from build123d import *

# Parameters (mm, degrees)
SKETCH1_R           = 25
SKETCH1_R_2         = 10
SKETCH1_R_3         = 4
SKETCH1_R_4         = 20
BOSS_EXTRUDE1_DEPTH = 17.5
SKETCH1_4_R         = 25
SKETCH1_4_R_2       = 20
BOSS_EXTRUDE2_DEPTH = 27.5
SKETCH2_R           = 20
CUT_EXTRUDE1_DEPTH  = 12.5
CUT_EXTRUDE2_DEPTH  = 55.083893922
SKETCH1_5_R         = 10
SKETCH1_5_R_2       = 6
BOSS_EXTRUDE3_DEPTH = 21.5
FILLET3_R           = 15
CUT_EXTRUDE3_DEPTH  = 12.5
FILLET1_R           = 7.5
FILLET2_R           = 1.5


with BuildPart() as part:
    # Sketch1 → Boss-Extrude1 (new body, symmetric)
    with BuildSketch(Plane(origin=(0, 0, 0), x_dir=(1, 0, 0), z_dir=(0, 1, 0))):
        with BuildLine():
            ThreePointArc((23.169245136, -48.74831039), (44.696355929, -24.926018406), (75, -14.314362055))
            Line((75, -14.314362055), (171.881275704, -5.838348723))
            ThreePointArc((171.881275704, -5.838348723), (170, 0), (171.881275704, 5.838348723))
            Line((171.881275704, 5.838348723), (75, 14.314362055))
            ThreePointArc((75, 14.314362055), (44.696355929, 24.926018406), (23.169245136, 48.74831039))
            ThreePointArc((23.169245136, 48.74831039), (24.030815541, 46.486476164), (24.323725422, 44.083893922))
            ThreePointArc((24.323725422, 44.083893922), (11.593351964, 34.463859578), (5.814713266, 49.337151209))
            ThreePointArc((5.814713266, 49.337151209), (-11.588137289, 35.664619361), (-33.70385172, 36.496791078))
            ThreePointArc((-33.70385172, 36.496791078), (-29.194535449, 32.814838368), (-27.5, 27.2453448))
            ThreePointArc((-27.5, 27.2453448), (-34.054404214, 17.857700278), (-45.125573936, 20.776139119))
            ThreePointArc((-45.125573936, 20.776139119), (-37.5, 0), (-45.125573936, -20.776139119))
            ThreePointArc((-45.125573936, -20.776139119), (-34.054404214, -17.857700278), (-27.5, -27.2453448))
            ThreePointArc((-27.5, -27.2453448), (-29.194535449, -32.814838368), (-33.70385172, -36.496791078))
            ThreePointArc((-33.70385172, -36.496791078), (-11.588137289, -35.664619361), (5.814713266, -49.337151209))
            ThreePointArc((5.814713266, -49.337151209), (11.593351964, -34.463859578), (24.323725422, -44.083893922))
            ThreePointArc((24.323725422, -44.083893922), (24.030815541, -46.486476164), (23.169245136, -48.74831039))
        make_face()
        Circle(SKETCH1_R, mode=Mode.SUBTRACT)
        with Locations((14.323725422, 44.083893922)):
            Circle(SKETCH1_R_2)
        with Locations((14.323725422, 44.083893922)):
            Circle(SKETCH1_R_3, mode=Mode.SUBTRACT)
        with Locations((-37.5, 27.2453448)):
            Circle(SKETCH1_R_2)
        with Locations((-37.5, 27.2453448)):
            Circle(SKETCH1_R_3, mode=Mode.SUBTRACT)
        with Locations((-37.5, -27.2453448)):
            Circle(SKETCH1_R_2)
        with Locations((-37.5, -27.2453448)):
            Circle(SKETCH1_R_3, mode=Mode.SUBTRACT)
        with Locations((14.323725422, -44.083893922)):
            Circle(SKETCH1_R_2)
        with Locations((14.323725422, -44.083893922)):
            Circle(SKETCH1_R_3, mode=Mode.SUBTRACT)
        Circle(SKETCH1_R)
        Circle(SKETCH1_R_4, mode=Mode.SUBTRACT)
    extrude(amount=BOSS_EXTRUDE1_DEPTH, both=True)

    # Sketch1_4 → Boss-Extrude2 (add, symmetric)
    with BuildSketch(Plane(origin=(0, 0, 0), x_dir=(1, 0, 0), z_dir=(0, 1, 0))):
        Circle(SKETCH1_4_R)
        Circle(SKETCH1_4_R_2, mode=Mode.SUBTRACT)
    extrude(amount=BOSS_EXTRUDE2_DEPTH, both=True)

    # Sketch2 → Cut-Extrude1 (cut, symmetric)
    with BuildSketch(Plane(origin=(0, 0, 0), x_dir=(1, 0, 0), z_dir=(0, 1, 0))):
        Circle(SKETCH2_R)
        with BuildLine():
            ThreePointArc((9.905954739, 28.31734558), (-30, 0), (9.905954739, -28.31734558))
            ThreePointArc((9.905954739, -28.31734558), (42.01613595, -19.285159783), (75, -14.314362055))
            ThreePointArc((75, -14.314362055), (44.696355929, -24.926018406), (23.169245136, -48.74831039))
            ThreePointArc((23.169245136, -48.74831039), (14.662831175, -54.078142632), (5.814713266, -49.337151209))
            ThreePointArc((5.814713266, -49.337151209), (-11.588137289, -35.664619361), (-33.70385172, -36.496791078))
            ThreePointArc((-33.70385172, -36.496791078), (-45.590169944, -33.123197323), (-45.125573936, -20.776139119))
            ThreePointArc((-45.125573936, -20.776139119), (-37.5, 0), (-45.125573936, 20.776139119))
            ThreePointArc((-45.125573936, 20.776139119), (-45.590169944, 33.123197323), (-33.70385172, 36.496791078))
            ThreePointArc((-33.70385172, 36.496791078), (-11.588137289, 35.664619361), (5.814713266, 49.337151209))
            ThreePointArc((5.814713266, 49.337151209), (14.662831175, 54.078142632), (23.169245136, 48.74831039))
            ThreePointArc((23.169245136, 48.74831039), (44.696355929, 24.926018406), (75, 14.314362055))
            ThreePointArc((75, 14.314362055), (42.01613595, 19.285159783), (9.905954739, 28.31734558))
        make_face()
    extrude(amount=CUT_EXTRUDE1_DEPTH, both=True, mode=Mode.SUBTRACT)

    # Sketch3 → Cut-Extrude2 (cut, symmetric)
    with BuildSketch(Plane.XY):
        with BuildLine():
            Line((171.881275704, 17.5), (171.881275704, 9.5))
            Line((171.881275704, 9.5), (119.899888641, 9.5))
            ThreePointArc((119.899888641, 9.5), (97.096380139, 11.515625954), (75, 17.5))
            Line((75, 17.5), (119.899888641, 17.5))
            Line((119.899888641, 17.5), (171.881275704, 17.5))
        make_face()
    cut_extrude2 = extrude(amount=CUT_EXTRUDE2_DEPTH, both=True, mode=Mode.SUBTRACT)

    # Mirror1: Cut-Extrude2 across plane
    add(cut_extrude2.mirror(Plane.ZX), mode=Mode.SUBTRACT)

    # Sketch1_5 → Boss-Extrude3 (add, symmetric)
    with BuildSketch(Plane(origin=(0, 0, 0), x_dir=(1, 0, 0), z_dir=(0, 1, 0))):
        with Locations((180, 0)):
            Circle(SKETCH1_5_R)
        with Locations((180, 0)):
            Circle(SKETCH1_5_R_2, mode=Mode.SUBTRACT)
    extrude(amount=BOSS_EXTRUDE3_DEPTH, both=True)

    # Fillet3
    fillet3_edges = [part.edges().sort_by_distance(p)[0] for p in [
        (171.881275704, 0, -5.838348723),
        (171.881275704, 0, 5.838348723),
    ]]
    fillet(fillet3_edges, radius=FILLET3_R)

    # Sketch4 → Cut-Extrude3 (cut)
    with BuildSketch(Plane(origin=(0, 17.5, 0), x_dir=(1, 0, 0), z_dir=(0, 1, 0))):
        with BuildLine():
            Line((65, 10.672059421), (65, -10.672059421))
            Line((65, -10.672059421), (119.507687799, -5.903254663))
            Line((119.507687799, -5.903254663), (165.620941154, -1.868867757))
            ThreePointArc((165.620941154, -1.868867757), (165.5, 0), (165.620941154, 1.868867757))
            Line((165.620941154, 1.868867757), (119.507687799, 5.903254663))
            Line((119.507687799, 5.903254663), (65, 10.672059421))
        make_face()
    cut_extrude3 = extrude(amount=-CUT_EXTRUDE3_DEPTH, mode=Mode.SUBTRACT)

    # Mirror2: Cut-Extrude3 across plane
    add(cut_extrude3.mirror(Plane.ZX), mode=Mode.SUBTRACT)

    # Fillet1
    fillet1_edges = [part.edges().sort_by_distance(p)[0] for p in [
        (65, 11.25, -10.672059421),
        (65, 11.25, 10.672059421),
        (65, -11.25, -10.672059421),
        (65, -11.25, 10.672059421),
    ]]
    fillet(fillet1_edges, radius=FILLET1_R)

    # Fillet2
    fillet2_edges = [part.edges().sort_by_distance(p)[0] for p in [
        (165.620941154, 7.25, -1.868867757),
        (165.620941154, 7.25, 1.868867757),
        (165.620941154, -7.25, 1.868867757),
        (165.620941154, -7.25, -1.868867757),
    ]]
    fillet(fillet2_edges, radius=FILLET2_R)


solid = part.part
CAD build for the part. Positions are in the model's coordinates, mm. A direction names the side the tool comes from. Coordinates: 2 decimals unless noted, no trailing zeros. Write each loop counter-clockwise with the first axis right and the second up, starting at its lowest first coordinate (ties: lowest second). Pieces come first, ordered by that corner, then holes. Notation, with made-up numbers: M 32.25,88 L 62.25,88 A27 ccw 62.25,114 Z; hole C -10,54 d5. An arc over 180 degrees is marked long. Answer as a JSON object with one key per item and string values. Group by question number.
1) Saw through at A-A (x = 180). Write the cut outline in (y, z), plus the area to 3 significant figures.
2) Mould opens along X. For faces 1 (the face through (14.81, -14.965, -54.072)), 2 (the face through (170.45, 0.13, 6.74)), 3 (the face through (97.41, -11.46, -10.03)), 4 (the face through (-37.5, 15, -0.3)) say: +X half, -X half, draft (parallel to the pull), parting line (faces both ways), or undercut.
3) Saw through at B-B (y = 0). Write the cut outline in (x, z).
4) Tool access for faces 5 (the face through (-27, 12.5, -16)), 6 (the face through (23.846, -22.43, -7.509)), 7 (the face through (42.473, 0.175, -19.187)): list every direction of +Z, -Z, +X, -X, +Y, -Y with a clear straight run to the whole face (end or side of a thin tool).
5) Wall check: line 1 (Z direction, x = -37, y = -16); line 2 (X direction, y = -1.5, z = -0.5); line 3 (Z direction, x = 180, y = 5). Give the ranges that are in metal, low to high. Write a range as from..to.
6) Saw through at D-D (x = 0). Write the cut outline in (y, z), plus the area to 3 significant figures.
7) Pin check, flat tips, straight feed: pin 1 Ø24 at (x, z) = (0, 0) entering from -Y; pin 2 Ø2 at (x, y) = (153.5, -6.5) entering from -Z; pin 3 Ø22 at (x, z) = (177.5, 2) entering from +Y; pin 4 Ø6 at (x, y) = (39.5, 4) entering from -Z. Stop position of each tip, or through.
8) Saw through at C-C (x = 32.5). Write the cut outline in (y, z).
Values follow:
{
 "1": {"outline": "M -21.5,-10 L 21.5,-10 L 21.5,-6 L -21.5,-6 Z; M -21.5,6 L 21.5,6 L 21.5,10 L -21.5,10 Z", "area": "344 mm2"},
 "2": {"face 1": "parting line", "face 2": "undercut", "face 3": "undercut", "face 4": "-X half"},
 "3": {"outline": "M 9.91,-28.32 A267.83 cw 75,-14.31 L 165.65,-6.38 A15 cw 174.78,-8.53 A10 ccw long 174.78,8.53 A15 cw 165.65,6.38 L 75,14.31 A267.83 cw 9.91,28.32 A30 ccw long Z; hole C 0,0 d40; hole C 180,0 d12"},
 "4": {"face 5": "none", "face 6": "-Y", "face 7": "-Z, +X"},
 "5": {"line 1": "z = -37.23..-31.21, -23.28..23.28, 31.21..37.23", "line 2": "x = -30..-19.99, 19.99..174.02, 185.98..189.99", "line 3": "z = -10..-6, 6..10"},
 "6": {"outline": "M -27.5,-25 L -17.5,-25 L -17.5,-42.36 L -12.5,-42.36 L -12.5,-30 L 12.5,-30 L 12.5,-42.36 L 17.5,-42.36 L 17.5,-25 L 27.5,-25 L 27.5,-20 L -27.5,-20 Z; M -27.5,20 L 27.5,20 L 27.5,25 L 17.5,25 L 17.5,42.36 L 12.5,42.36 L 12.5,30 L -12.5,30 L -12.5,42.36 L -17.5,42.36 L -17.5,25 L -27.5,25 Z", "area": "1,150 mm2"},
 "7": {"pin 1": "passes through", "pin 2": "stops at z = -7.53", "pin 3": "stops at y = 21.5", "pin 4": "stops at z = -20.53"},
 "8": {"outline": "M -17.5,-35.42 L -12.5,-35.42 L -12.5,-21.51 L 12.5,-21.51 L 12.5,-35.42 L 17.5,-35.42 L 17.5,35.42 L 12.5,35.42 L 12.5,21.51 L -12.5,21.51 L -12.5,35.42 L -17.5,35.42 Z"}
}
